The model under review builds one solid part; all positions refer to its coordinate system, in mm. Face numbers are marked on the shaded views. Give positions to 0.01 mm unless a question says otherwise; leave off trailing zeros. Write each loop counter-clockwise with the first axis right and the second up, starting at its lowest first coordinate (ties: lowest second). Pieces come first, ordered by that corner, then holes.
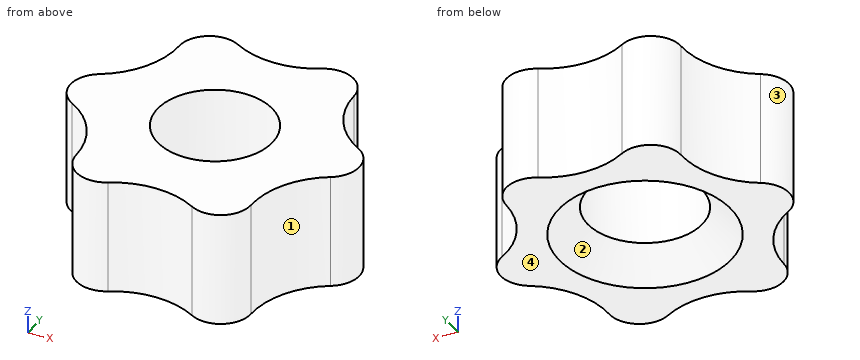
Autodesk Inventor part; units mm, degrees
ref_plane "YZ Plane" through (0, 0, 0) normal (1, 0, 0) x (0, 1, 0)
ref_plane "XZ Plane" through (0, 0, 0) normal (0, 1, 0) x (-1, 0, 0)
ref_plane "XY Plane" through (0, 0, 0) normal (0, 0, 1) x (1, 0, 0)
sketch "スケッチ1" plane through (0, 0, 0) normal (0, 0, 1) x (1, 0, 0)
  arc A0 (144.025, 105.9095) -> (145.475, 108.4209) centre (142.575, 108.4209) ccw
  arc A1 (145.475, 101.5793) -> (144.025, 104.0908) centre (142.575, 101.5793) ccw
  line L0 (146, 100.67) -> (143.5, 105.0001) construction
  arc A2 (144.025, 105.9095) -> (144.025, 104.0908) centre (144.55, 105.0001) ccw
  line L1 (143.5, 105.0001) -> (146, 109.3303) construction
  circle A3 centre (148.5, 105.0001) radius 5 construction
  arc A4 (149.95, 100.67) -> (147.05, 100.67) centre (148.5, 98.1585) ccw
  line L2 (151, 100.67) -> (146, 100.67) construction
  arc A5 (145.475, 101.5793) -> (147.05, 100.67) centre (146.525, 101.5793) ccw
  arc A6 (149.95, 100.67) -> (151.525, 101.5793) centre (150.475, 101.5793) ccw
  arc A7 (152.975, 104.0908) -> (151.525, 101.5793) centre (154.425, 101.5793) ccw
  line L3 (153.5, 105.0001) -> (151, 100.67) construction
  arc A8 (152.975, 104.0908) -> (152.975, 105.9095) centre (152.45, 105.0001) ccw
  circle A9 centre (148.5, 105.0001) radius 2
  line L4 (151, 109.3303) -> (153.5, 105.0001) construction
  arc A10 (151.525, 108.4209) -> (152.975, 105.9095) centre (154.425, 108.4209) ccw
  arc A11 (151.525, 108.4209) -> (149.95, 109.3303) centre (150.475, 108.4209) ccw
  line L5 (146, 109.3303) -> (151, 109.3303) construction
  arc A12 (147.05, 109.3303) -> (149.95, 109.3303) centre (148.5, 111.8417) ccw
  arc A13 (147.05, 109.3303) -> (145.475, 108.4209) centre (146.525, 108.4209) ccw
  circle A14 centre (148.5, 105.0001) radius 6 construction
  point P0 (0, 0)
  point P1 (146, 100.67)
  point P2 (151, 100.67)
  point P3 (153.5, 105.0001)
  point P4 (145.475, 101.5793)
  point P5 (151.525, 101.5793)
  point P6 (152.975, 104.0908)
  point P7 (152.975, 105.9095)
  point P8 (151.525, 108.4209)
  point P9 (145.475, 108.4209)
  point P10 (144.025, 105.9095)
  point P11 (144.025, 104.0908)
  dimension "d4" = 10
  dimension "d5" = 360
  dimension "d6" = 360
  dimension "d7" = 1.05
  dimension "d8" = 4
  dimension "d9" = 12
extrude "押し出し1" add sketch "スケッチ1" along normal blind 4
chamfer "面取り1" distance 1 angle 45 1 edges at (146.5, 105.0001, 0)
properties part number "3ギア接続部3" material "アルミニウム 2014-T4"
1) Consider section A-A, the plane x = 148.5. Give the boundary of the cut face in (y, z), then the cut area to 3 significant figures.
2) To check wall thickness, follow probe 1 along Y at (x, z) = (148.5, 3.1); probe 2 along Y at (x, z) = (149.75, 3.1) (3 decimals); probe 3 along X at (y, z) = (105.25, 0.75). State the ranges of each line that lie inside material, in increasing order.
3) Insertion check: pin 1 (1.5 mm diameter, centred on x = 149.5, z = 1, fed in from +Y); pin 2 (1 mm diameter, centred on x = 147.5, z = 1, fed in from -Y). Each pin has a flat end and moves straight along its axis. Give the tip position at first contact, or say it passes through.
4) Consider section D-D, the plane y = 108.75. Give the boundary of the cut face in (x, z).
5) The part is to be moulded in two halves that separate along X. For the marked faces 1, 2, 3 and 4, say which applies: +X half, -X half, draft (parallel to the pull), parting line (faces both ways), or undercut.
Answer block:
1. outline: (101.06, 0) - (102, 0) - (103, 1) - (103, 4) - (101.06, 4) - close; (107, 1) - (108, 0) - (108.94, 0) - (108.94, 4) - (107, 4) - close
1. area: 14.5 mm2
2. probe 1: y = 101.06 to 103, 107 to 108.94
2. probe 2: y = 100.775 to 103.439, 106.561 to 109.225
2. probe 3: x = 143.53 to 146.26, 150.74 to 153.47
3. pin 1: stops at y = 109.45
3. pin 2: stops at y = 100.64
4. outline: (145.53, 0) - (151.47, 0) - (151.47, 4) - (145.53, 4) - close
5. face 1: +X half
5. face 2: undercut
5. face 3: -X half
5. face 4: draft
